CAD build for the part. Positions are in the model's coordinates, mm. Face numbers are marked on the shaded views. A direction names the side the tool comes from. Round coordinates to 2 decimals unless told otherwise and drop trailing zeros. Order: outer loops, then holes, each group sorted by start corner. A loop starts at its lowest first (then second) coordinate and runs counter-clockwise, first axis right, second up. Notation, with made-up numbers: (42.5, 35) - (78.5, 35) arc R12 cw to (78.5, 46) - close; hole circle Ø3 at (-7, -22.75). An arc over 180 degrees is marked (long way). Use one line per item in the form item = value. Start each with the question number.
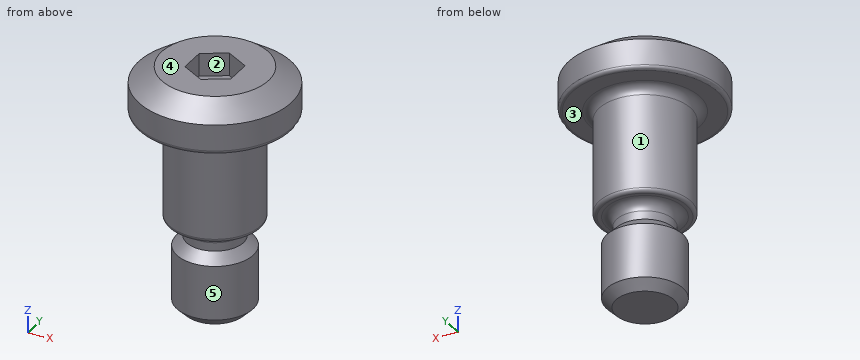
from build123d import *

# Parameters (mm, degrees)
CUT_EXTRUDE2_DEPTH = 1.5
CHAMFER1_SIZE      = 0.6
CHAMFER2_SIZE      = 1.5
CHAMFER2_SIZE2     = 1.050311307
FILLET1_R          = 0.24
FILLET2_R          = 0.6


with BuildPart() as part:
    # Sketch10 → Revolve1 (revolve)
    with BuildSketch(Plane(origin=(0, 0, 0), x_dir=(0, 0, -1), z_dir=(1, 0, 0))):
        Polygon((10, 3), (10, 2.5), (16, 2.5), (16, 0), (0, 0), (0, 5), (3, 5), (3, 3), align=None)
    revolve(axis=Axis((0, 0, -16), (0, 0, 1)))

    # Sketch5 → Cut-Revolve1 (revolve, cut)
    with BuildSketch(Plane(origin=(0, 0, 0), x_dir=(0, 0, -1), z_dir=(1, 0, 0))):
        with BuildLine():
            Line((10, 3), (12.345, 3))
            Line((12.345, 3), (11.2, 1.855))
            Line((11.2, 1.855), (10.645, 1.855))
            ThreePointArc((10.645, 1.855), (10.188916126, 2.043916126), (10, 2.5))
            Line((10, 2.5), (10, 3))
        make_face()
    revolve(axis=Axis((0, 0, -16), (0, 0, 1)), mode=Mode.SUBTRACT)

    # Sketch8 → Cut-Extrude2 (cut)
    with BuildSketch(Plane.XY):
        Polygon((0, 1.732050808), (-1.5, 0.866025404), (-1.5, -0.866025404), (0, -1.732050808), (1.5, -0.866025404), (1.5, 0.866025404), align=None)
    extrude(amount=-CUT_EXTRUDE2_DEPTH, mode=Mode.SUBTRACT)

    # Chamfer1
    chamfer1_edges = [part.edges().sort_by_distance(p)[0] for p in [
        (0, -2.5, -16),
    ]]
    chamfer(chamfer1_edges, length=CHAMFER1_SIZE)

    # Chamfer2
    chamfer2_edges = [part.edges().sort_by_distance(p)[0] for p in [
        (0, -5, 0),
    ]]
    chamfer2_side = [part.faces().sort_by_distance(p)[0] for p in [
        (0, -4.858578644, 0),
    ]]
    chamfer(chamfer2_edges, length=CHAMFER2_SIZE, length2=CHAMFER2_SIZE2, reference=chamfer2_side[0])

    # Fillet1
    fillet1_edges = [part.edges().sort_by_distance(p)[0] for p in [
        (0, -5, -3),
        (0, -3, -10),
    ]]
    fillet(fillet1_edges, radius=FILLET1_R)

    # Fillet2
    fillet2_edges = [part.edges().sort_by_distance(p)[0] for p in [
        (0, -3, -3),
    ]]
    fillet(fillet2_edges, radius=FILLET2_R)


solid = part.part
(1) Slice it at C-C (z = -15). Give the cut face in (x, y), and give its area (3 significant figures).
(2) Slice it at B-B (z = -6). Give the cut face in (x, y).
(3) Which spindle directions (+Z, -Z, +X, -X, +Y, -Y) get a long thin tool onto all of the face, cutting with end or side? Do the marked faces 4 and 5. Say none if no direction does.
(4) Flat gauge pins, fed straight in: P1, Ø1.5, axis at x = -3.5, z = -6, coming from the +Y side; P2, Ø5, axis at x = 2.5, z = -6.5, coming from the -Y side; P3, Ø5, axis at y = -2.5, z = -6.5, coming from the -X side. Where does each tip first touch, or does it go through?
(5) Mould opens along X. For the marked faces 1, 2 and 3 say: pulls with the +X half, pulls with the -X half, needs draft (parallel to the pull), parting line crosses it, or undercut.
(6) Wall check: line 1 (Z direction, x = 1, y = 0.5); line 2 (Y direction, x = -1, z = -0.75); line 3 (Z direction, x = 2.5, y = 1). Give the ranges that are in metal, low to high. Write a range as [from, to].
Results list:
q1.outline = circle Ø5 at (0, 0)
q1.area = 19.6 mm²
q2.outline = circle Ø6 at (0, 0)
q3.face_4 = +Z, +X, -X, +Y, -Y
q3.face_5 = -Z
q4.P1 = 1.2
q4.P2 = -3
q4.P3 = -3
q5.face_1 = parting line crosses it
q5.face_2 = undercut
q5.face_3 = needs draft
q6.line_1 = [-16, -1.5]
q6.line_2 = [-4.46, -1.15], [1.15, 4.46]
q6.line_3 = [-10, 0]
